Part model, mm, in its own coordinate system. Face numbers are marked on the shaded views. A direction names the side the tool comes from. Coordinates: 2 decimals unless noted, no trailing zeros. Loops run counter-clockwise (first coordinate to the right, second up) from the corner with the lowest first, then second, coordinate; pieces in that order, holes last. Notation, with made-up numbers: M 23,49.25 L 53,49.25 A21 ccw 53,80.25 Z; hole C -36.5,27.25 d2. An arc over 180 degrees is marked long. Answer as a JSON object with one key per item and string values. Group by question number.
1. Drill centre lines: L1, parallel to Y at x = -16, z = 16; L2, parallel to X at y = -6.5, z = 9.5; L3, parallel to Z at x = -3.5, y = -7. Where is each one in solid material? Low to high.
2. Saw through at C-C on x = -14. Write the cut outline in (y, z), then the cut area to 3 significant figures.
3. Drop flat-ended pins along their axis: pin 1 Ø14.5 at (x, y) = (1.5, 31.5) entering from +Z; pin 2 Ø4 at (y, z) = (31.33, -21.75) entering from +X; pin 3 Ø3 at (x, z) = (-5.5, -5) entering from -Y; pin 4 Ø4 at (x, y) = (4, 31.5) entering from +Z. Give the stop position or say it passes through.
4. 3-axis set-ups, long thin cutter, end or side, ignore diameter. For the marked faces 5, 6 and 7: which of +Z, -Z, +X, -X, +Y, -Y reach the whole face in a straight line?
5. Saw through at A-A on z = -21.75. Count the separate pieces of the cut face and the enclosed holes in it, then the cut area to 4 significant figures.
6. Mould opens along Y. For the marked faces 1, 2, 3 and 4 say: released by +Y, released by -Y, zero draft, split by the parting line, or undercut.
7. Saw through at B-B on y = -8.5. Write the cut outline in (x, z), then the cut area to 3 significant figures.
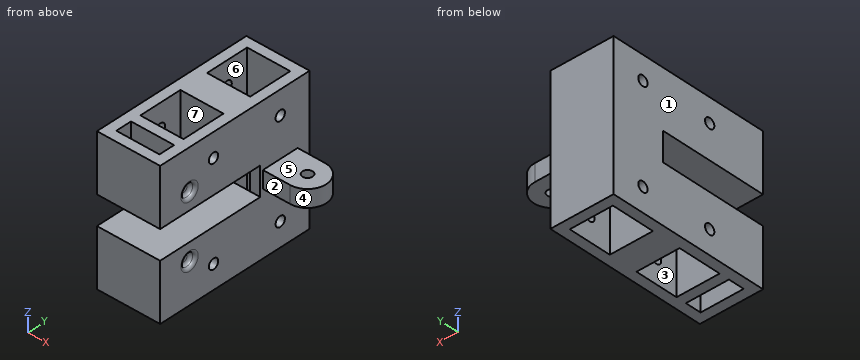
from build123d import *

# Parameters (mm, degrees)
SKETCH1_W                = 22
SKETCH1_H                = 56
SKETCH1_W_2              = 15
SKETCH1_H_2              = 15
BOSS_EXTRUDE1_DEPTH      = 20
SKETCH2_W                = 15
SKETCH2_H                = 15
SKETCH2_H_2              = 5.5
CUT_EXTRUDE1_DEPTH       = 15.5
SKETCH3_R                = 1.75
CUT_EXTRUDE2_DEPTH       = 35
BOSS_EXTRUDE2_DEPTH      = 10
BOSS_EXTRUDE3_DEPTH      = 3
BOSS_EXTRUDE3_DEPTH_BACK = 3
SKETCH6_R                = 1.75
SKETCH7_R                = 2.25
CUT_EXTRUDE3_DEPTH       = 2
FILLET1_R                = 1


with BuildPart() as part:
    # Sketch1 → Boss-Extrude1 (new body)
    with BuildSketch(Plane.XY):
        with Locations((-14.096172604, 14.333947726)):
            Rectangle(SKETCH1_W, SKETCH1_H)
        with Locations((-14.096172604, 31.333947726)):
            Rectangle(SKETCH1_W_2, SKETCH1_H_2, mode=Mode.SUBTRACT)
    extrude(amount=BOSS_EXTRUDE1_DEPTH)

    # Sketch2 → Cut-Extrude1 (cut)
    with BuildSketch(Plane.XY.offset(20)):
        with Locations((-14.096172604, 6.333947726)):
            Rectangle(SKETCH2_W, SKETCH2_H)
        with Locations((-14.096172604, -7.416052274)):
            Rectangle(SKETCH2_W, SKETCH2_H_2)
    extrude(amount=-CUT_EXTRUDE1_DEPTH, mode=Mode.SUBTRACT)

    # Sketch3 → Cut-Extrude2 (cut)
    with BuildSketch(Plane.ZY.offset(25.096172604)):
        with Locations(Location((11.75, 31.333947726, 0), (0, 0, 270))):
            Circle(SKETCH3_R)
        with Locations(Location((11.75, 6.333947726, 0), (0, 0, 90))):
            Circle(SKETCH3_R)
    extrude(amount=-CUT_EXTRUDE2_DEPTH, mode=Mode.SUBTRACT)


with BuildPart() as body_2:
    # Mirror3: mirrored copy
    add(part.part.mirror(Plane(origin=(0, 0, -5), x_dir=(1, 0, 0), z_dir=(0, 0, -1))))


with BuildPart() as part_1:
    add(part.part)

    add(body_2.part)  # Boss-Extrude2 merges body 2
    # Sketch4 → Boss-Extrude2 (add)
    with BuildSketch(Plane(origin=(0, 0, 0), x_dir=(-1, 0, 0), z_dir=(0, 0, -1))):
        Polygon((6.596172604, 38.833947726), (21.596172604, 38.833947726), (21.596172604, 23.833947726), (25.096172604, 23.833947726), (25.096172604, 42.333947726), (3.096172604, 42.333947726), (3.096172604, 23.833947726), (6.596172604, 23.833947726), align=None)
    extrude(amount=BOSS_EXTRUDE2_DEPTH)

    # Sketch6 → Boss-Extrude3 (add, two sides: drawn at the far end of the back side and taken through both)
    with BuildSketch(Plane(origin=(0, 0, -5), x_dir=(-1, 0, 0), z_dir=(0, 0, -1)).offset(-BOSS_EXTRUDE3_DEPTH_BACK)):
        with BuildLine():
            Line((-6.403827396, 37.833947726), (3.096172604, 37.833947726))
            Line((3.096172604, 37.833947726), (3.096172604, 24.833947726))
            Line((3.096172604, 24.833947726), (-6.403827396, 24.833947726))
            ThreePointArc((-6.403827396, 24.833947726), (-12.903827396, 31.333947726), (-6.403827396, 37.833947726))
        make_face()
        with Locations((-6.403827396, 31.333947726)):
            Circle(SKETCH6_R, mode=Mode.SUBTRACT)
    extrude(amount=BOSS_EXTRUDE3_DEPTH + BOSS_EXTRUDE3_DEPTH_BACK)

    # Sketch7 → Cut-Extrude3 (cut)
    with BuildSketch(Plane(origin=(-3.096172604, 0, 0), x_dir=(0, 0, -1), z_dir=(1, 0, 0))):
        with Locations(Location((16, -2.666052274, 0), (0, 0, 90))):
            Circle(SKETCH7_R)
        with Locations(Location((-6, -2.666052274, 0), (0, 0, 90))):
            Circle(SKETCH7_R)
    extrude(amount=-CUT_EXTRUDE3_DEPTH, mode=Mode.SUBTRACT)

    # Fillet1
    fillet1_edges = [part_1.edges().sort_by_distance(p)[0] for p in [
        (-5.096172604, -4.916052274, -16),
        (-3.096172604, -4.916052274, -16),
        (-5.096172604, -4.916052274, 6),
        (-3.096172604, -4.916052274, 6),
    ]]
    fillet(fillet1_edges, radius=FILLET1_R - 0.0001)  # a hair under: the kernel refuses the full size


solid = part_1.part
Outcome:
{
 "1": {"L1": "y = -13.67 to -10.17, -4.67 to -1.17, 13.83 to 23.83, 38.83 to 42.33", "L2": "x = -25.1 to -21.6, -6.6 to -3.1", "L3": "z = -30 to -10, 0 to 20"},
 "2": {"outline": "M -13.67,-30 L -10.17,-30 L -10.17,-14.5 L -4.67,-14.5 L -4.67,-30 L -1.17,-30 L -1.17,-14.5 L 13.83,-14.5 L 13.83,-30 L 23.83,-30 L 23.83,-10 L -13.67,-10 Z; M -13.67,0 L 23.83,0 L 23.83,20 L 13.83,20 L 13.83,4.5 L -1.17,4.5 L -1.17,20 L -4.67,20 L -4.67,4.5 L -10.17,4.5 L -10.17,20 L -13.67,20 Z; M 38.83,-30 L 42.33,-30 L 42.33,20 L 38.83,20 Z", "area": "1,040 mm²"},
 "3": {"pin 1": "stops at z = 20", "pin 2": "stops at x = -3.1", "pin 3": "stops at y = 23.83", "pin 4": "stops at z = -2"},
 "4": {"face 5": "+Z, +X, +Y, -Y", "face 6": "+Z, -Z", "face 7": "+Z"},
 "5": {"separate pieces": "3", "enclosed holes": "1", "area": "650.5 mm²"},
 "6": {"face 1": "zero draft", "face 2": "released by -Y", "face 3": "undercut", "face 4": "split by the parting line"},
 "7": {"outline": "M -25.1,-30 L -21.6,-30 L -21.6,-14.5 L -6.6,-14.5 L -6.6,-30 L -3.1,-30 L -3.1,-10 L -25.1,-10 Z; M -25.1,0 L -3.1,0 L -3.1,20 L -6.6,20 L -6.6,4.5 L -21.6,4.5 L -21.6,20 L -25.1,20 Z", "area": "415 mm²"}
}
